Could you check a few things on this model? Use its own coordinates, in mm. A direction names the side the tool comes from. Coordinates: 2 decimals unless noted, no trailing zeros. Loops run counter-clockwise (first coordinate to the right, second up) from the corner with the lowest first, then second, coordinate; pieces in that order, holes last.
from build123d import *

# Parameters (mm, degrees)
F0_R     = 53.95
F1_DEPTH = 4.763
F2_D     = 6.7564


with BuildPart() as f1:
    # F0 (on Top) → F1 (new body)
    with BuildSketch(Plane.XY):
        Circle(F0_R)
        with BuildLine():
            ThreePointArc((38.1, -12.7), (36.2401280605, -17.1901280605), (31.75, -19.05))
            Line((31.75, -19.05), (-31.75, -19.05))
            ThreePointArc((-31.75, -19.05), (-36.2401280605, -17.1901280605), (-38.1, -12.7))
            Line((-38.1, -12.7), (-38.1, 12.7))
            ThreePointArc((-38.1, 12.7), (-36.2401280605, 17.1901280605), (-31.75, 19.05))
            Line((-31.75, 19.05), (31.75, 19.05))
            ThreePointArc((31.75, 19.05), (36.2401280605, 17.1901280605), (38.1, 12.7))
            Line((38.1, 12.7), (38.1, -12.7))
        make_face(mode=Mode.SUBTRACT)
    extrude(amount=F1_DEPTH)

    # F2 (through all)
    with Locations(Plane(origin=(0, 0, 0), x_dir=(1, 0, 0), z_dir=(0, 0, -1))):
        with Locations((33.9453681376, -33.9453681376), (-33.9453681376, -33.9453681376), (-33.9453681376, 33.9453681376), (33.9453681376, 33.9453681376)):
            Hole(F2_D / 2)


solid = f1.part
1) Imagine slicing it at B-B on x = 0. List the corners of the cut face in (y, z) for me.
2) If I drill on L1, parallel to X at y = 32, z = 1.25; L2, parallel to Y at x = 0, z = 3.7; L3, parallel to Y at x = -31, z = 3, over which ranges is the centre line in solid material (lowest first)?
3) Will these pins go through, and if not, where does the flat tip stop? pin 1 (1.4 mm diameter, centred on y = -1.5, z = 2.5, fed in from +X); pin 2 (1 mm diameter, centred on x = -20.5, z = 1, fed in from -Y); pin 3 (1 mm diameter, centred on x = 17, z = 3.5, fed in from +Y); pin 4 (10 mm diameter, centred on x = 13.5, y = 10.5, fed in from +Z).
4) Imagine slicing it at C-C on z = 3.55. List the corners of the cut face in (x, y) for me.
5) For faces 1 (the flat face through (-1, -23, 0)), 2 (the cylindrical face through (36.29, -17.14, 2.35)), which set-ups out of +Z, -Z, +X, -X, +Y, -Y let a thin tool reach every point of the face, with its end or its side?
6) Imagine slicing it at A-A on y = 0. List the corners of the cut face in (x, z) for me.
7) We'd pull the mould along X, two halves only. Please class faces 3 (the cylindrical face through (-53.898, 2.372, 2.348)), 4 (the flat face through (38.1, 0, 2)), 5 (the flat face through (-1, -23, 4.763)): released by +X, released by -X, zero draft, split by the parting line, or undercut.
8) Imagine slicing it at D-D on x = 33. List the corners of the cut face in (y, z) for me.
Solved:
1. outline: (-53.95, 0) - (-19.05, 0) - (-19.05, 4.76) - (-53.95, 4.76) - close; (19.05, 0) - (53.95, 0) - (53.95, 4.76) - (19.05, 4.76) - close
2. L1: x = -43.44 to -36.71, -31.18 to 31.18, 36.71 to 43.44
2. L2: y = -53.95 to -19.05, 19.05 to 53.95
2. L3: y = -44.15 to -35.6, -32.29 to -19.05, 19.05 to 32.29, 35.6 to 44.15
3. pin 1: stops at x = 53.94
3. pin 2: stops at y = -50.11
3. pin 3: stops at y = 51.36
3. pin 4: passes through
4. outline: circle Ø107.9 at (0, 0); hole (-38.1, -12.7) arc R6.35 ccw to (-31.75, -19.05) - (31.75, -19.05) arc R6.35 ccw to (38.1, -12.7) - (38.1, 12.7) arc R6.35 ccw to (31.75, 19.05) - (-31.75, 19.05) arc R6.35 ccw to (-38.1, 12.7) - close; hole circle Ø6.76 at (-33.95, -33.95); hole circle Ø6.76 at (-33.95, 33.95); hole circle Ø6.76 at (33.95, -33.95); hole circle Ø6.76 at (33.95, 33.95)
5. face 1: -Z, +X, -X, +Y, -Y
5. face 2: +Z, -Z
6. outline: (-53.95, 0) - (-38.1, 0) - (-38.1, 4.76) - (-53.95, 4.76) - close; (38.1, 0) - (53.95, 0) - (53.95, 4.76) - (38.1, 4.76) - close
7. face 3: split by the parting line
7. face 4: undercut
7. face 5: zero draft
8. outline: (-42.68, 0) - (-37.19, 0) - (-37.19, 4.76) - (-42.68, 4.76) - close; (-30.7, 0) - (-18.93, 0) - (-18.93, 4.76) - (-30.7, 4.76) - close; (18.93, 0) - (30.7, 0) - (30.7, 4.76) - (18.93, 4.76) - close; (37.19, 0) - (42.68, 0) - (42.68, 4.76) - (37.19, 4.76) - close
